Input: part model. Units: mm. Frame: model coordinates. A direction names the side the tool comes from. Give positions to 0.01 mm unless a question says otherwise; leave off trailing zeros. Loops run counter-clockwise (first coordinate to the right, second up) from the corner with the lowest first, then second, coordinate; pieces in that order, holes last. Notation, with made-up numbers: (31.5, 89.5) -> (86.5, 89.5) arc R30 ccw to (86.5, 118.5) -> close; hole circle Ø5 at (6.25, 4.25). An arc over 180 degrees is marked (long way). Answer as a JSON object with one key per item and string values. Group by question number.
```python
from build123d import *

# Parameters (mm, degrees)
SKETCH_1_W          = 54.8
SKETCH_1_H          = 54.8
SKETCH_1_R          = 12.5
SKETCH_1_R_2        = 1.6
SKETCH_1_W_2        = 4.4
SKETCH_1_H_2        = 8
SKETCH_1_W_3        = 8
SKETCH_1_H_3        = 4.4
EXTRUDE_1_DEPTH     = 4.4
FILLET_1_R          = 6
SKETCH_2_R          = 1.6
CUT_EXTRUDE_1_DEPTH = 10


with BuildPart() as part:
    # 草图1 → 凸台-拉伸1 (new body)
    with BuildSketch(Plane(origin=(0, 0, 0), x_dir=(1, 0, 0), z_dir=(0, 1, 0))):
        Rectangle(SKETCH_1_W, SKETCH_1_H)
        Circle(SKETCH_1_R, mode=Mode.SUBTRACT)
        with Locations((21.4, 21.4)):
            Circle(SKETCH_1_R_2, mode=Mode.SUBTRACT)
        with Locations((21.4, -21.4)):
            Circle(SKETCH_1_R_2, mode=Mode.SUBTRACT)
        with Locations((-21.4, -21.4)):
            Circle(SKETCH_1_R_2, mode=Mode.SUBTRACT)
        with Locations((-21.4, 21.4)):
            Circle(SKETCH_1_R_2, mode=Mode.SUBTRACT)
        with Locations((20.2, 9)):
            Rectangle(SKETCH_1_W_2, SKETCH_1_H_2, mode=Mode.SUBTRACT)
        with Locations((20.2, -9)):
            Rectangle(SKETCH_1_W_2, SKETCH_1_H_2, mode=Mode.SUBTRACT)
        with Locations((-20.2, -9)):
            Rectangle(SKETCH_1_W_2, SKETCH_1_H_2, mode=Mode.SUBTRACT)
        with Locations((-20.2, 9)):
            Rectangle(SKETCH_1_W_2, SKETCH_1_H_2, mode=Mode.SUBTRACT)
        with Locations((9, 20.2)):
            Rectangle(SKETCH_1_W_3, SKETCH_1_H_3, mode=Mode.SUBTRACT)
        with Locations((9, -20.2)):
            Rectangle(SKETCH_1_W_3, SKETCH_1_H_3, mode=Mode.SUBTRACT)
        with Locations((-9, -20.2)):
            Rectangle(SKETCH_1_W_3, SKETCH_1_H_3, mode=Mode.SUBTRACT)
        with Locations((-9, 20.2)):
            Rectangle(SKETCH_1_W_3, SKETCH_1_H_3, mode=Mode.SUBTRACT)
    extrude(amount=EXTRUDE_1_DEPTH)

    # 圆角1
    fillet_1_edges = [part.edges().sort_by_distance(p)[0] for p in [
        (27.4, 2.2, 27.4),
        (-27.4, 2.2, 27.4),
        (-27.4, 2.2, -27.4),
        (27.4, 2.2, -27.4),
    ]]
    fillet(fillet_1_edges, radius=FILLET_1_R)

    # 草图2 → 切除-拉伸1 (cut)
    with BuildSketch(Plane(origin=(0, 4.4, 0), x_dir=(1, 0, 0), z_dir=(0, 1, 0))):
        with Locations((10.7, 10.7)):
            Circle(SKETCH_2_R)
        with Locations((10.7, -10.7)):
            Circle(SKETCH_2_R)
        with Locations((-10.7, -10.7)):
            Circle(SKETCH_2_R)
        with Locations((-10.7, 10.7)):
            Circle(SKETCH_2_R)
    extrude(amount=-CUT_EXTRUDE_1_DEPTH, mode=Mode.SUBTRACT)


solid = part.part
```
Q1. Pull-direction query (X, two-part tool) for faces 3 (the face through (0, 2, -27.4)), 4 (the face through (25.596, 2.231, -25.689)), 5 (the face through (-13, 2, 20)); classes: +X half, -X half, draft (parallel to the pull), parting line (faces both ways), or undercut.
Q2. Ray query, probe 1 along X at (y, z) = (3.4, 21.4); probe 2 along Z at (x, y) = (-10.7, 1.9). Return the intervals inside material, ascending.
Q3. Section A-A on x = 7.5. Return the cut outline in (y, z).
Q4. Section C-C on z = -10.7. Return the cut outline in (x, y).
Q5. Section D-D on y = 1.6. State how many separate pieces and enclosed holes the cut face has, then the cut area to 3 significant figures.
Q6. Set-up query: faces 1 (the face through (-20, 2, -5)), 2 (the face through (12, 0, 6)). Return all of +Z, -Z, +X, -X, +Y, -Y with unobstructed straight access to the full face (end or side cutting, diameter ignored); none if empty.
Q7. Pin query (flat end, axial travel): pin 1 Ø4 at (x, z) = (-7, 7) entering from +Y; pin 2 Ø5 at (x, z) = (-21.4, 21.4) entering from +Y. Return the tip coordinate at first contact, or that it passes through.
Q8. Section B-B on z = 0. Return the cut outline in (x, y).
Numbers:
{
 "1": {"face 3": "draft", "face 4": "+X half", "face 5": "undercut"},
 "2": {"probe 1": "x = -27.4 to -23, -19.8 to -13, -5 to 5, 13 to 19.8, 23 to 27.4", "probe 2": "z = -27.4 to -22.4, -18 to -12.3, -9.1 to -6.46, 6.46 to 9.1, 12.3 to 18, 22.4 to 27.4"},
 "3": {"outline": "(0, -27.4) -> (4.4, -27.4) -> (4.4, -22.4) -> (0, -22.4) -> close; (0, -18) -> (4.4, -18) -> (4.4, -10) -> (0, -10) -> close; (0, 10) -> (4.4, 10) -> (4.4, 18) -> (0, 18) -> close; (0, 22.4) -> (4.4, 22.4) -> (4.4, 27.4) -> (0, 27.4) -> close"},
 "4": {"outline": "(-27.4, 0) -> (-22.4, 0) -> (-22.4, 4.4) -> (-27.4, 4.4) -> close; (-18, 0) -> (-12.3, 0) -> (-12.3, 4.4) -> (-18, 4.4) -> close; (-9.1, 0) -> (-6.46, 0) -> (-6.46, 4.4) -> (-9.1, 4.4) -> close; (6.46, 0) -> (9.1, 0) -> (9.1, 4.4) -> (6.46, 4.4) -> close; (12.3, 0) -> (18, 0) -> (18, 4.4) -> (12.3, 4.4) -> close; (22.4, 0) -> (27.4, 0) -> (27.4, 4.4) -> (22.4, 4.4) -> close"},
 "5": {"separate pieces": "1", "enclosed holes": "17", "area": "2,140 mm²"},
 "6": {"face 1": "+Y, -Y", "face 2": "+Z, -Z, +X, -X, -Y"},
 "7": {"pin 1": "passes through", "pin 2": "stops at y = 4.4"},
 "8": {"outline": "(-27.4, 0) -> (-12.5, 0) -> (-12.5, 4.4) -> (-27.4, 4.4) -> close; (12.5, 0) -> (27.4, 0) -> (27.4, 4.4) -> (12.5, 4.4) -> close"}
}
